Study the drawing (mm; zero at the part's minimum x, y, z) and answer. Coordinates: 2 decimals unless noted, no trailing zeros. Loops run counter-clockwise (first coordinate to the right, second up) from the corner with the lowest first, then second, coordinate; pieces in that order, holes last. Notation, with made-up numbers: (-13.75, -23) - (20.25, -23) arc R12 cw to (20.25, -17) - close; hole circle Ø8 at (-29.75, -11). An arc over 180 degrees is marked (long way). Use CSV: the item, a comma, the result in double quotes.
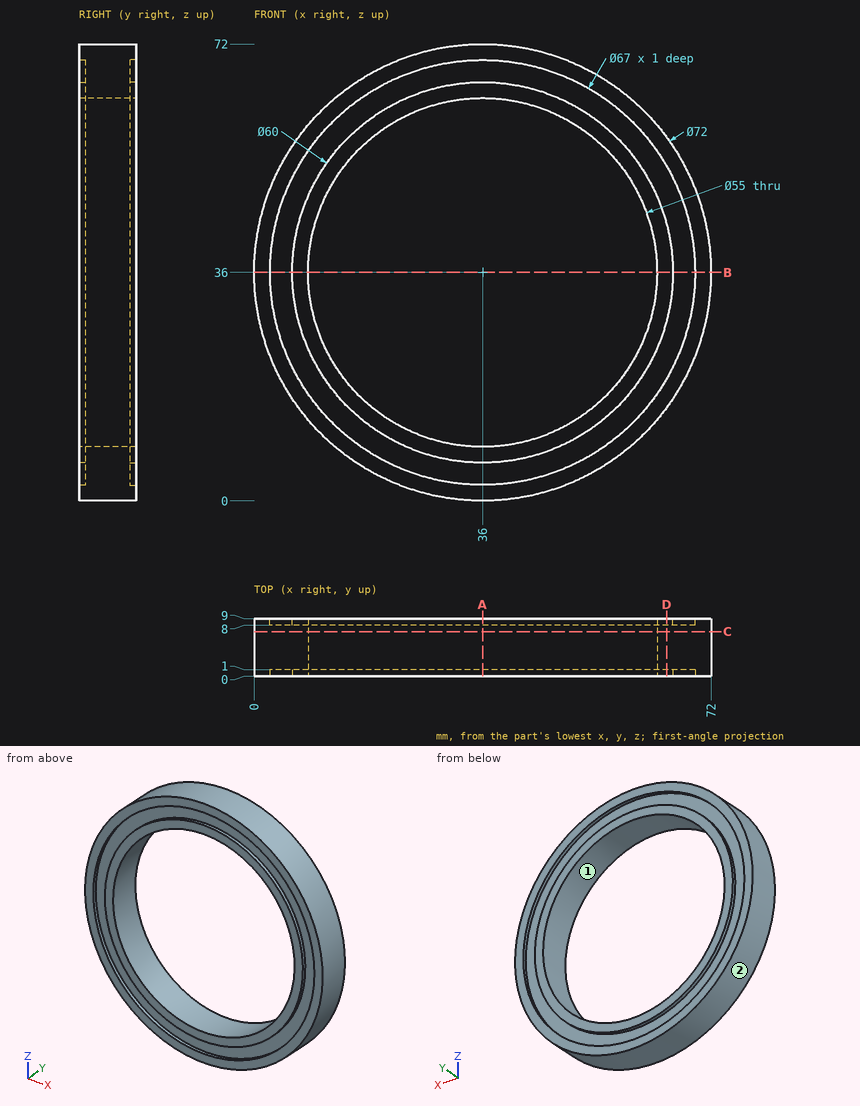
Q1. The part is cut by section A-A on x = 36. Determine the outline of the cut face in (y, z), and give its area (3 significant figures).
Reported:
outline,"(0, 0) - (9, 0) - (9, 2.5) - (8, 2.5) - (8, 6) - (9, 6) - (9, 8.5) - (0, 8.5) - (0, 6) - (1, 6) - (1, 2.5) - (0, 2.5) - close; (0, 63.5) - (9, 63.5) - (9, 66) - (8, 66) - (8, 69.5) - (9, 69.5) - (9, 72) - (0, 72) - (0, 69.5) - (1, 69.5) - (1, 66) - (0, 66) - close"
area,"139 mm²"
Q2. Find the intervals of material crossed by probe 1 along X at (y, z) = (0.6, 36); probe 2 along X at (y, z) = (6.25, 36); probe 3 along Z at (x, y) = (26.5, 8.75), in increasing order. Write a range as [from, to].
Reported:
probe 1,"x = [0, 2.5], [6, 8.5], [63.5, 66], [69.5, 72]"
probe 2,"x = [0, 8.5], [63.5, 72]"
probe 3,"z = [1.28, 3.88], [7.54, 10.19], [61.81, 64.46], [68.12, 70.72]"
Q3. The part is cut by section C-C on y = 7. Determine the outline of the cut face in (x, z), and give its area (3 significant figures).
Reported:
outline,"circle Ø72 at (36, 36); hole circle Ø55 at (36, 36)"
area,"1,700 mm²"
Q4. For a pull along X with two mould halves and no side action, classify the marked faces 1 and 2 as +X half, -X half, draft (parallel to the pull), parting line (faces both ways), or undercut.
Reported:
face 1,"undercut"
face 2,"parting line"
Q5. Given P1, Ø5, axis at y = 7.5, z = 43, coming from the +X side; P2, Ø1.5, axis at y = 5.5, z = 8, coming from the +X side; P3, Ø4, axis at x = 56.5, y = 5, coming from the -Z side, each flat-ended and moving along its own axis, determine where each tip first touches the part or whether it passes through.
Reported:
P1,"stops at x = 71.72"
P2,"stops at x = 59.53"
P3,"stops at z = 5.12"
Q6. The part is cut by section B-B on z = 36. Determine the outline of the cut face in (x, y).
Reported:
outline,"(0, 0) - (2.5, 0) - (2.5, 1) - (6, 1) - (6, 0) - (8.5, 0) - (8.5, 9) - (6, 9) - (6, 8) - (2.5, 8) - (2.5, 9) - (0, 9) - close; (63.5, 0) - (66, 0) - (66, 1) - (69.5, 1) - (69.5, 0) - (72, 0) - (72, 9) - (69.5, 9) - (69.5, 8) - (66, 8) - (66, 9) - (63.5, 9) - close"
Q7. The part is cut by section D-D on x = 65. Determine the outline of the cut face in (y, z).
Reported:
outline,"(0, 14.67) - (9, 14.67) - (9, 19.23) - (8, 19.23) - (8, 28.32) - (9, 28.32) - (9, 43.68) - (8, 43.68) - (8, 52.77) - (9, 52.77) - (9, 57.33) - (0, 57.33) - (0, 52.77) - (1, 52.77) - (1, 43.68) - (0, 43.68) - (0, 28.32) - (1, 28.32) - (1, 19.23) - (0, 19.23) - close"
